from build123d import *

# Parameters (mm, degrees)
F1_DEPTH = 4.318
F2_R     = 5.08


with BuildPart() as f1:
    # F0 (on Top) → F1 (new body)
    with BuildSketch(Plane.XY):
        Polygon((-32.902525, -8.854119), (-36.682051, -5.389552), (-36.682051, 4.689189), (43.317949, 4.689189), (43.317949, -5.389552), (39.538425, -8.854119), (48.357325, -12.318687), (48.357325, 10.043521), (-41.721424, 10.043521), (-41.721424, -12.318687), align=None)
    extrude(amount=F1_DEPTH)

    # F2
    f2_edges = [f1.edges().sort_by_distance(p)[0] for p in [
        (-36.682051, 4.689189, 2.159),
        (43.317949, 4.689189, 2.159),
        (-36.682051, -5.389552, 2.159),
        (43.317949, -5.389552, 2.159),
    ]]
    fillet(f2_edges, radius=F2_R)


solid = f1.part
Part model, mm, in its own coordinate system. A direction names the side the tool comes from. Give positions to 0.01 mm unless a question says otherwise; leave off trailing zeros. Loops run counter-clockwise (first coordinate to the right, second up) from the corner with the lowest first, then second, coordinate; pieces in that order, holes last. Notation, with made-up numbers: (70, 4.25) -> (117, 4.25) arc R32 cw to (117, 41.25) -> close; hole circle Ø5 at (-10.75, 51). An arc over 180 degrees is marked (long way). Write each question's results on one line, items separated by ' | '. Start each with the question number.
Q1. Wall check: L1, parallel to X at y = -0.25, z = 4.1; L2, parallel to X at y = 3, z = 2.2; L3, parallel to Y at x = 19.5, z = 1.8. Give the ranges that are in metal, low to high.
Q2. Pin check, flat tip, straight feed: P1, Ø2, axis at x = -30, z = 3, coming from the -Y side. Stop position of the tip, or through.
Q3. Band-saw the part on B-B on z = 1.5. List the corners of the cut face in (x, y), plus the area to 3 significant figures.
Q4. Which spindle directions (+Z, -Z, +X, -X, +Y, -Y) get a long thin tool onto all of the face, cutting with end or side? Do faces 5 (the face through (40.62, -7.86, 2.13)), 6 (the face through (3, 4.689, 2)), 7 (the face through (3, 5, 0)). Say none if no direction does.
Q5. Band-saw the part on D-D on y = -6. List the corners of the cut face in (x, z), plus the area to 3 significant figures.
Q6. Pull direction Y, two halves, no side cores. Call faces 1 (the face through (-36.682, -2, 2)), 2 (the face through (-41.721, -1, 2)), 3 (the face through (4, 10.044, 2)), 4 (the face through (43.886, -10.562, 2.129)): +Y half, -Y half, draft (parallel to the pull), parting line (faces both ways), or undercut.
Q7. Band-saw the part on C-C on x = 4. List the corners of the cut face in (y, z), plus the area to 3 significant figures.
Q8. Band-saw the part on A-A on y = 3. List the corners of the cut face in (x, z), plus the area to 3 significant figures.
Results are:
1) L1: x = -41.72 to -36.68, 43.32 to 48.36 | L2: x = -41.72 to -35.38, 42.02 to 48.36 | L3: y = 4.69 to 10.04
2) P1: stops at y = 4.69
3) outline: (-41.72, -12.32) -> (-32.9, -8.85) -> (-35.03, -6.9) arc R5.08 cw to (-36.68, -3.15) -> (-36.68, -0.39) arc R5.08 cw to (-31.6, 4.69) -> (38.24, 4.69) arc R5.08 cw to (43.32, -0.39) -> (43.32, -3.15) arc R5.08 cw to (41.67, -6.9) -> (39.54, -8.85) -> (48.36, -12.32) -> (48.36, 10.04) -> (-41.72, 10.04) -> close | area: 675 mm²
4) face 5: +Z, -Z | face 6: +Z, -Z, -Y | face 7: -Z, +X, -X, +Y, -Y
5) outline: (-41.72, 0) -> (-35.81, 0) -> (-35.81, 4.32) -> (-41.72, 4.32) -> close; (42.45, 0) -> (48.36, 0) -> (48.36, 4.32) -> (42.45, 4.32) -> close | area: 51.0 mm²
6) face 1: undercut | face 2: draft | face 3: +Y half | face 4: -Y half
7) outline: (4.69, 0) -> (10.04, 0) -> (10.04, 4.32) -> (4.69, 4.32) -> close | area: 23.1 mm²
8) outline: (-41.72, 0) -> (-35.38, 0) -> (-35.38, 4.32) -> (-41.72, 4.32) -> close; (42.02, 0) -> (48.36, 0) -> (48.36, 4.32) -> (42.02, 4.32) -> close | area: 54.7 mm²
